Part model, mm, in its own coordinate system. Give positions to 0.01 mm unless a question says otherwise; leave off trailing zeros. Write each loop counter-clockwise with the first axis right and the second up, starting at its lowest first coordinate (ties: lowest second). Pieces come first, ordered by that corner, then holes. Notation, with made-up numbers: (-28.75, -35.75) - (19.25, -35.75) arc R11 cw to (19.25, -18.75) - close; hole circle Ø5 at (17, 43). An arc over 180 degrees is marked (long way). Answer as a JSON object with one key per item and string values. Group by question number.
```python
from build123d import *

# Parameters (mm, degrees)
SKETCH1_W           = 254
SKETCH1_H           = 5.08
BOSS_EXTRUDE1_DEPTH = 203.2
SKETCH3_R           = 6.35
CUT_EXTRUDE1_DEPTH  = 6.08
SKETCH5_R           = 1.5875
CUT_EXTRUDE2_DEPTH  = 152.4
SKETCH12_R          = 3.175
CUT_EXTRUDE7_DEPTH  = 6.08
SKETCH14_R          = 3.175
CUT_EXTRUDE8_DEPTH  = 5.08
CUT_EXTRUDE9_REACH  = 7.08
SKETCH15_W          = 254
SKETCH15_H          = 10.16
SKETCH16_R          = 3.175
CUT_EXTRUDE10_DEPTH = 6.08
SKETCH19_R          = 3.175
CUT_EXTRUDE11_DEPTH = 5.08


with BuildPart() as part:
    # Sketch1 → Boss-Extrude1 (new body)
    with BuildSketch(Plane.XY):
        Rectangle(SKETCH1_W, SKETCH1_H)
    extrude(amount=BOSS_EXTRUDE1_DEPTH)

    # Sketch3 → Cut-Extrude1 (cut, through all)
    with BuildSketch(Plane(origin=(0, 2.54, 0), x_dir=(1, 0, 0), z_dir=(0, 1, 0))):
        with Locations((-114.3, -22.86)):
            Circle(SKETCH3_R)
        with Locations((-114.3, -180.34)):
            Circle(SKETCH3_R)
        with Locations((114.3, -22.86)):
            Circle(SKETCH3_R)
        with Locations((114.3, -180.34)):
            Circle(SKETCH3_R)
    extrude(amount=-CUT_EXTRUDE1_DEPTH, mode=Mode.SUBTRACT)

    # Sketch5 → Cut-Extrude2 (cut)
    with BuildSketch(Plane(origin=(0, 2.54, 0), x_dir=(1, 0, 0), z_dir=(0, 1, 0))):
        with Locations((97.63, -133.2)):
            Circle(SKETCH5_R)
        with Locations((97.63, -145.9)):
            Circle(SKETCH5_R)
        with Locations((-19.21, -133.2)):
            Circle(SKETCH5_R)
        with Locations((-19.21, -145.9)):
            Circle(SKETCH5_R)
        with Locations((-97.696, -133.2)):
            Circle(SKETCH5_R)
        with Locations((-97.696, -145.9)):
            Circle(SKETCH5_R)
        with Locations((19.144, -133.2)):
            Circle(SKETCH5_R)
        with Locations((19.144, -145.9)):
            Circle(SKETCH5_R)
    extrude(amount=-CUT_EXTRUDE2_DEPTH, mode=Mode.SUBTRACT)

    # Sketch12 → Cut-Extrude7 (cut, through all)
    with BuildSketch(Plane(origin=(0, 2.54, 0), x_dir=(1, 0, 0), z_dir=(0, 1, 0))):
        with Locations((-90.0557, -29.21)):
            Circle(SKETCH12_R)
        with Locations((-42.6212, -29.21)):
            Circle(SKETCH12_R)
    cut_extrude7 = extrude(amount=-CUT_EXTRUDE7_DEPTH, mode=Mode.SUBTRACT)

    # Sketch14 → Cut-Extrude8 (cut)
    with BuildSketch(Plane(origin=(0, 2.54, 0), x_dir=(1, 0, 0), z_dir=(0, 1, 0))):
        with Locations((-32.832800096, -16.51)):
            Circle(SKETCH14_R)
        with Locations((-32.832800096, -41.91)):
            Circle(SKETCH14_R)
    cut_extrude8 = extrude(amount=-CUT_EXTRUDE8_DEPTH, mode=Mode.SUBTRACT)

    # Mirror1: Cut-Extrude7, Cut-Extrude8 across plane
    add(cut_extrude7.mirror(Plane(origin=(0, 0, 0), x_dir=(0, 0, 1), z_dir=(1, 0, 0))), mode=Mode.SUBTRACT)
    add(cut_extrude8.mirror(Plane(origin=(0, 0, 0), x_dir=(0, 0, 1), z_dir=(1, 0, 0))), mode=Mode.SUBTRACT)

    # Sketch15 → Cut-Extrude9 (cut, up to next)
    with BuildSketch(Plane(origin=(0, 2.54, 0), x_dir=(1, 0, 0), z_dir=(0, 1, 0)), mode=Mode.PRIVATE) as cut_extrude9_sk1:
        with Locations((0, -5.08)):
            Rectangle(SKETCH15_W, SKETCH15_H)
    cut_extrude9_tool1 = extrude(cut_extrude9_sk1.sketch, amount=-CUT_EXTRUDE9_REACH, mode=Mode.PRIVATE) & part.part
    add(cut_extrude9_tool1.solids().sort_by_distance((0, 2.54, 5.08))[0], mode=Mode.SUBTRACT)

    # Sketch16 → Cut-Extrude10 (cut, through all)
    with BuildSketch(Plane(origin=(0, 2.54, 0), x_dir=(1, 0, 0), z_dir=(0, 1, 0))):
        with Locations((84.0486, -196.85)):
            Circle(SKETCH16_R)
        with Locations((84.0486, -171.45)):
            Circle(SKETCH16_R)
    cut_extrude10 = extrude(amount=-CUT_EXTRUDE10_DEPTH, mode=Mode.SUBTRACT)

    # Mirror2: Cut-Extrude10 across plane
    add(cut_extrude10.mirror(Plane(origin=(0, 0, 0), x_dir=(0, 0, 1), z_dir=(1, 0, 0))), mode=Mode.SUBTRACT)

    # Sketch19 → Cut-Extrude11 (cut)
    with BuildSketch(Plane(origin=(0, 2.54, 0), x_dir=(1, 0, 0), z_dir=(0, 1, 0))):
        with Locations((-28.357399872, -171.45)):
            Circle(SKETCH19_R)
        with Locations((-28.357399872, -196.85)):
            Circle(SKETCH19_R)
    cut_extrude11 = extrude(amount=-CUT_EXTRUDE11_DEPTH, mode=Mode.SUBTRACT)

    # Mirror3: Cut-Extrude11 across plane
    add(cut_extrude11.mirror(Plane(origin=(0, 0, 0), x_dir=(0, 0, 1), z_dir=(1, 0, 0))), mode=Mode.SUBTRACT)


solid = part.part
```
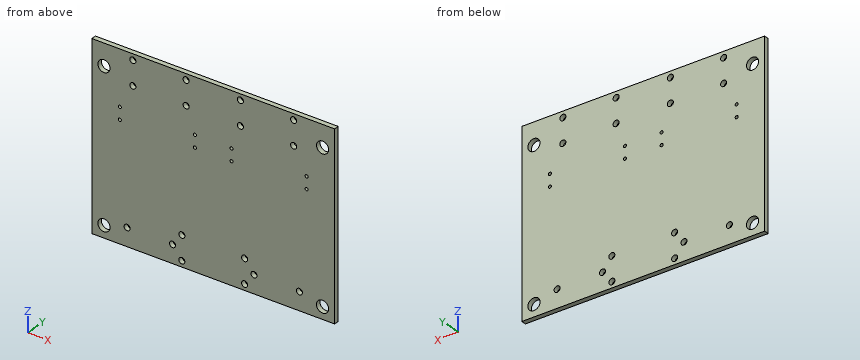
1) Probe line 1 (Z direction, x = 114.3, y = 0.7); line 2 (X direction, y = 1.35, z = 180.34); line 3 (X direction, y = -1.05, z = 41.91). List the from-to ranges inside material, lowest first.
2) Band-saw the part on C-C (x = -42.5). List the corners of the cut face in (y, z), plus the area to 3 significant figures.
3) Band-saw the part on B-B (z = 196.85). List the corners of the cut face in (x, y), plus the area to 3 significant figures.
4) Band-saw the part on A-A (y = 0.7). State how many separate pieces and enclosed holes the cut face has, plus the area to 3 significant figures.
5) Drop a flat-ended pin along its axis: P1, Ø5, axis at x = -19.21, z = 133.2, coming from the +Y side. Give the stop position or say it passes through.
Verdict:
{
 "1": {"line 1": "10.16 to 16.51, 29.21 to 173.99, 186.69 to 203.2", "line 2": "-127 to -120.65, -107.95 to 107.95, 120.65 to 127", "line 3": "-127 to -36.01, -29.66 to 29.66, 36.01 to 127"},
 "2": {"outline": "(-2.54, 10.16) - (2.54, 10.16) - (2.54, 26.04) - (-2.54, 26.04) - close; (-2.54, 32.38) - (2.54, 32.38) - (2.54, 203.2) - (-2.54, 203.2) - close", "area": "948 mm2"},
 "3": {"outline": "(-127, -2.54) - (-87.22, -2.54) - (-87.22, 2.54) - (-127, 2.54) - close; (-80.87, -2.54) - (-31.53, -2.54) - (-31.53, 2.54) - (-80.87, 2.54) - close; (-25.18, -2.54) - (25.18, -2.54) - (25.18, 2.54) - (-25.18, 2.54) - close; (31.53, -2.54) - (80.87, -2.54) - (80.87, 2.54) - (31.53, 2.54) - close; (87.22, -2.54) - (127, -2.54) - (127, 2.54) - (87.22, 2.54) - close", "area": "1,160 mm2"},
 "4": {"separate pieces": "1", "enclosed holes": "28", "area": "48,000 mm2"},
 "5": {"P1": "y = 2.54"}
}
